Geometry: final body of the model. Coordinates: model frame, mm. A direction names the side the tool comes from. Give positions to 0.01 mm unless a question says otherwise; leave off trailing zeros. Order: outer loops, then holes, each group sorted by start corner. A loop starts at its lowest first (then second) coordinate and runs counter-clockwise, first axis right, second up. Notation, with made-up numbers: (-16.75, 86) -> (-1.75, 86) arc R23 ccw to (-1.75, 119) -> close; hole circle Ø4 at (-15, 22). An arc over 180 degrees is marked (long way). One line per item, written item: value. Start each with the question number.
```python
from build123d import *

# Parameters (mm, degrees)
CORTAR_EXTRUIR1_DEPTH      = 10
CORTAR_EXTRUIR1_DEPTH_BACK = 10
CROQUIS3_W                 = 10.64526068670476
CROQUIS3_H                 = 3.3994785725990075
CROQUIS4_R                 = 2.000000000000003
CORTAR_EXTRUIR2_DEPTH      = 10
CORTAR_EXTRUIR3_DEPTH      = 12


with BuildPart() as part:
    # Croquis1 → Revoluci_n1 (revolve)
    with BuildSketch(Plane(origin=(0, 0, 0), x_dir=(1, 0, 0), z_dir=(0, 1, 0))):
        with BuildLine():
            Line((0, 0), (-14, 0))
            ThreePointArc((-14, 0), (-7.000000000000001, -7), (0, 0))
        make_face()
    revolve(axis=Axis((0, 0, 0), (-1, 0, 0)))

    # Croquis2 → Revoluci_n2 (revolve)
    with BuildSketch(Plane(origin=(0, 0, 0), x_dir=(1, 0, 0), z_dir=(0, 1, 0)), mode=Mode.PRIVATE) as revoluci_n2_sk:
        with BuildLine():
            Line((-14, 0), (-63, -7.72e-15))
            ThreePointArc((-63, -7.72e-15), (-59.08463499046059, -4.880939145028195), (-53.47057322501258, -2.117614953202559))
            ThreePointArc((-53.47057322501258, -2.117614953202559), (-53.239158217402505, -2.028995288641408), (-52.99305737642324, -2.0000000000000018))
            Line((-52.99305737642324, -2.0000000000000018), (-17.584352216063312, -2.0000000000000018))
            ThreePointArc((-17.584352216063312, -2.0000000000000018), (-15.254449379168335, -2.3517694688151263), (-13.132252927177912, -3.3757182994316812))
            Line((-13.132252927177912, -3.3757182994316812), (-14, 0))
        make_face()
    revolve(revoluci_n2_sk.sketch.rotate(Axis((0, 0, 0), (-1, 0, 0)), 180), axis=Axis((0, 0, 0), (-1, 0, 0)))

    # Croquis3 → Cortar-Extruir1 (cut, two sides: drawn at the far end of the back side and taken through both)
    with BuildSketch(Plane(origin=(0, 0, 0), x_dir=(1, 0, 0), z_dir=(0, 1, 0)).offset(-CORTAR_EXTRUIR1_DEPTH_BACK)):
        with Locations((-58.793203568364966, 3.8173542395020648)):
            Rectangle(CROQUIS3_W, CROQUIS3_H)
        Polygon((-53.470573225012586, -2.1176149532025623), (-64.11583391171735, -2.1176149532025637), (-64.11583391171735, -5.334174428303361), (-53.470573225012586, -5.334174428303361), align=None)
    extrude(amount=CORTAR_EXTRUIR1_DEPTH + CORTAR_EXTRUIR1_DEPTH_BACK, mode=Mode.SUBTRACT)

    # Croquis4 → Cortar-Extruir2 (cut)
    with BuildSketch(Plane(origin=(0, 0, -2.117614953202561), x_dir=(-1, 0, 0), z_dir=(0, 0, -1))):
        with Locations((58, 0)):
            Circle(CROQUIS4_R)
    extrude(amount=-CORTAR_EXTRUIR2_DEPTH, mode=Mode.SUBTRACT)

    # Croquis5 → Cortar-Extruir3 (cut)
    with BuildSketch(Plane.XY.offset(2.1176149532025557)):
        with BuildLine():
            Line((-58, -3.2994521483388315), (-53.470573225012586, -2.1176149532025605))
            ThreePointArc((-53.470573225012586, -2.1176149532025605), (-63, -3.83e-15), (-53.470573225012586, 2.117614953202569))
            Line((-53.470573225012586, 2.117614953202569), (-58, 3.2994521483388315))
            ThreePointArc((-58, 3.2994521483388315), (-61.29945214833883, 4e-16), (-58, -3.2994521483388315))
        make_face()
    extrude(amount=-CORTAR_EXTRUIR3_DEPTH, mode=Mode.SUBTRACT)


solid = part.part
```
1. Material intervals for L1, parallel to Y at x = -58, z = -0.5; L2, parallel to Z at x = -57, y = -3; L3, parallel to Z at x = -40.5, y = -1.5, sorted ascending. Write a range as [from, to].
2. Cut plane B-B, the plane z = 5. Return loops of the section in (x, y).
3. Cut plane A-A, the plane x = -36. Return loops of the section in (y, z).
4. Pin query (flat end, axial travel): P1, Ø3.5, axis at x = -56, y = 0.5, coming from the +Z side; P2, Ø5, axis at x = -48.5, z = -2, coming from the -Y side; P3, Ø7.5, axis at x = -59, y = 1, coming from the -Z side. Return the tip coordinate at first contact, or that it passes through.
5. Access query for faces 1 (the flat face through (-55.6, 0, 2.118)), 2 (the flat face through (-55.767, -2.717, 0.03)), 3 (the cylindrical face through (-59.908, 0.601, -0.03)), 4 (the flat face through (-55.7, 2.7, 0)). Directions: +Z, -Z, +X, -X, +Y, -Y. A direction counts if a zero-diameter tool reaches every point of the face in a straight line with its end or side. Return the directions, or none.
6. Draft query along X for faces 5 (the cylindrical face through (-35, 1.2, 1.6)), 6 (the cylindrical face through (-61.3, 0.07, 0.03)), 7 (the flat face through (-55.7, 0, -2.118)). Return one class per face: pulls with the +X half, pulls with the -X half, needs draft (parallel to the pull), parting line crosses it, or undercut.
Answers follow:
1. L1: y = [-3.3, -2], [2, 3.3]
1. L2: z = [-2.12, 2.12]
1. L3: z = [-1.32, 1.32]
2. outline: circle Ø9.8 at (-7, 0)
3. outline: circle Ø4 at (0, 0)
4. P1: stops at z = 2.12
4. P2: stops at y = -2
4. P3: stops at z = -2.12
5. face 1: +Z, -X, +Y, -Y
5. face 2: +Z, -Z, -Y
5. face 3: +Z, -Z
5. face 4: +Z, -Z, +Y
6. face 5: undercut
6. face 6: pulls with the -X half
6. face 7: needs draft
